Input: dimensioned drawing with shaded views. Units: mm. Origin: part minimum x, y, z. A direction names the side the tool comes from. Round coordinates to 2 decimals unless told otherwise and drop trailing zeros. Order: outer loops, then holes, each group sorted by start corner. A loop starts at its lowest first (then second) coordinate and runs counter-clockwise, first axis right, second up. Notation, with made-up numbers: (-36.5, 29.25) - (5.5, 29.25) arc R38 cw to (5.5, 68.25) - close; hole circle Ø3 at (25, -12). An arc over 180 degrees is marked (long way). Return JSON: item names as keys, results as strings. Group by question number.
1) Contact query for flat-ended pins moving along their axis: P1, Ø3.5, axis at x = 36.5, y = 9, coming from the +Z side; P2, Ø3, axis at x = 51.5, y = 17.5, coming from the +Z side. Output: stop coordinate, or through.
2) Ray query, line 1 (Y direction, x = 11, z = 2.25); line 2 (X direction, y = 15, z = 1.5); line 3 (Y direction, x = 17.5, z = 0.8). Return the intervals inside material, ascending. Write a range as from..to.
3) Section B-B, the plane z = 5.25. Return loops of the section in (x, y), plus the area to 3 significant figures.
4) Section A-A, the plane x = 17.5. Return loops of the section in (y, z), plus the area to 3 significant figures.
5) Mould query, pull axis Y, two halves, no side actions, for the marked faces 1, 2 and 3. Classes: pulls with the +Y half, pulls with the -Y half, needs draft (parallel to the pull), parting line crosses it, or undercut.
6) Access query for the marked faces 4 and 5. Directions: +Z, -Z, +X, -X, +Y, -Y. A direction counts if a zero-diameter tool reaches every point of the face in a straight line with its end or side. Return the directions, or none.
7) Section D-D, the plane y = 22.75. Return loops of the section in (x, z).
8) Section C-C, the plane y = 15. Return loops of the section in (x, z), plus the area to 3 significant figures.
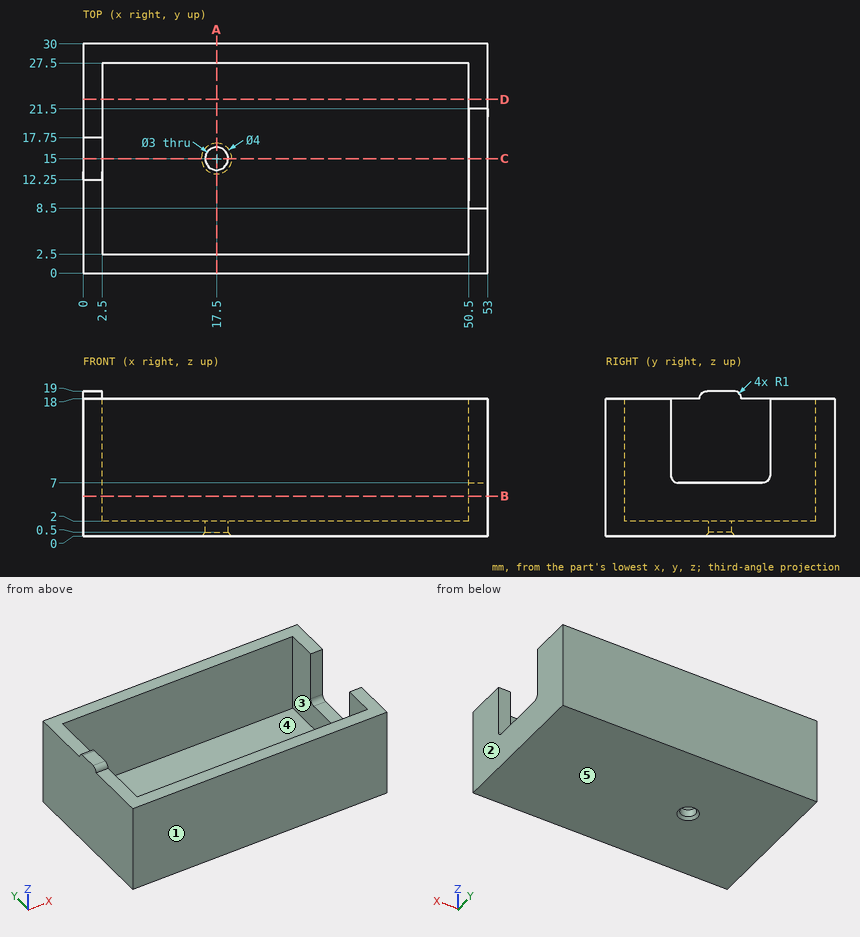
Geometry check:
{
 "1": {"P1": "z = 2", "P2": "z = 7"},
 "2": {"line 1": "0..2.5, 27.5..30", "line 2": "0..16, 19..53", "line 3": "0..13.5, 16.5..30"},
 "3": {"outline": "(0, 0) - (53, 0) - (53, 30) - (0, 30) - close; hole (2.5, 2.5) - (50.5, 2.5) - (50.5, 27.5) - (2.5, 27.5) - close", "area": "390 mm2"},
 "4": {"outline": "(0, 0) - (13, 0) - (13.5, 0.5) - (13.5, 2) - (2.5, 2) - (2.5, 18) - (0, 18) - close; (16.5, 0.5) - (17, 0) - (30, 0) - (30, 18) - (27.5, 18) - (27.5, 2) - (16.5, 2) - close", "area": "134 mm2"},
 "5": {"face 1": "pulls with the -Y half", "face 2": "needs draft", "face 3": "undercut"},
 "6": {"face 4": "+Z", "face 5": "-Z, +X, -X, +Y, -Y"},
 "7": {"outline": "(0, 0) - (53, 0) - (53, 18) - (50.5, 18) - (50.5, 2) - (2.5, 2) - (2.5, 18) - (0, 18) - close"},
 "8": {"outline": "(0, 0) - (15.5, 0) - (16, 0.5) - (16, 2) - (2.5, 2) - (2.5, 19) - (0, 19) - close; (19, 0.5) - (19.5, 0) - (53, 0) - (53, 7) - (50.5, 7) - (50.5, 2) - (19, 2) - close", "area": "155 mm2"}
}
